CAD build for the part. Positions are in the model's coordinates, mm. A direction names the side the tool comes from. Give positions to 0.01 mm unless a question says otherwise; leave off trailing zeros. Loops run counter-clockwise (first coordinate to the right, second up) from the corner with the lowest first, then second, coordinate; pieces in that order, holes last.
Item 1: Which spindle directions (+Z, -Z, +X, -X, +Y, -Y) get a long thin tool onto all of the face, cutting with end or side? Do faces 4 (the flat face through (0, 6, 3.175)), 5 (the flat face through (-4.21, -50.79, 16.19)). Say none if no direction does.
Item 2: Saw through at C-C on y = -45.5. Give the cut face in (x, z), plus the area to 3 significant figures.
Item 3: Saw through at A-A on y = -16.75. Give the cut face in (x, z) (3 decimals), plus the area to 3 significant figures.
Item 4: Drop flat-ended pins along their axis: P1, Ø4, axis at x = 2, y = -31, coming from the -Z side; P2, Ø3, axis at x = 0, y = 0, coming from the +Z side; P3, Ø4, axis at x = 2.5, y = -48.5, coming from the -Z side; P4, Ø1, axis at x = 1.5, z = 4.5, coming from the +Y side. Give the stop position or say it passes through.
Item 5: Saw through at B-B on x = 0. Give the number of separate pieces and of enclosed holes in the cut face, plus the area to 3 significant figures.
Item 6: Mould opens along X. For faces 1 (the flat face through (-6.5, -9, 3)), 2 (the cylindrical face through (-0.961, -48.552, 16.143)), 3 (the flat face through (-2, -42, 14.578)) say: released by +X, released by -X, zero draft, split by the parting line, or undercut.
Item 7: Probe probe 1 along X at (y, z) = (-45.5, 16.5); probe 2 along X at (y, z) = (16.75, 1.65); probe 3 along Y at (x, z) = (0, 0.6). List the from-to ranges inside material, lowest first.
Autodesk Inventor part; units mm, degrees
ref_plane "YZ Plane" through (0, 0, 0) normal (1, 0, 0) x (0, 1, 0)
ref_plane "XZ Plane" through (0, 0, 0) normal (0, 1, 0) x (-1, 0, 0)
ref_plane "XY Plane" through (0, 0, 0) normal (0, 0, 1) x (1, 0, 0)
sketch "Sketch1" plane through (0, 0, 0) normal (0, 0, 1) x (1, 0, 0)
  line L0 (6.5, -25) -> (-6.5, -25)
  line L1 (-6.5, -25) -> (-6.5, 25)
  line L2 (-6.5, 25) -> (6.5, 25)
  line L3 (6.5, 25) -> (6.5, -25)
  line L4 (6.5, -25) -> (-6.5, 25) construction
  line L5 (-6.5, -25) -> (6.5, 25) construction
  line L6 (0, 16.75) -> (0, -16.75) construction
  point P0 (0, 0)
  dimension "d0" = 50
  dimension "d1" = 13
  dimension "d2" = 33.5
extrude "Plate1" add sketch "Sketch1" along normal blind 3.175
hole "Hole1" at (0, 0, 0) at (0, 16.75, 0) at (0, -16.75, 0) direction (0, 0, 1) diameter 3.3 end through all
sketch "Sketch2" plane through (6.5, -27.7496, 4.7625) normal (0, -0.8660254, -0.5) x (1, 0, 0)
  line L0 (-13, 0) -> (0, 0)
  line L1 (0, 0) -> (0, 11.3338)
  line L2 (0, 11.3338) -> (-13, 11.3338)
  line L3 (-13, 11.3338) -> (-13, 0)
edge flange "Flange1" height 15 angle 60 thickness 3.175 bend radius 3.175 thickness toward (0, -0.8660254, -0.5) relief tear relief width 3.175 relief depth 1.5875 edges at (0, -25, 3.175) wall of the first edge with corners at (-6.5, -27.7496, 4.7625) (6.5, -27.7496, 4.7625) (6.5, -33.4165, 14.5779) (-6.5, -33.4165, 14.5779)
bend "Bend1"
corner "Corner1"
sketch "Sketch3" plane through (-6.5, -38.9158, 14.5779) normal (0, 0, 1) x (1, 0, 0)
  line L0 (13, 0) -> (0, 0)
  line L1 (0, 0) -> (0, -16.3338)
  line L2 (0, -16.3338) -> (13, -16.3338)
  line L3 (13, -16.3338) -> (13, 0)
edge flange "Flange2" height 20 angle 60 thickness 3.175 bend radius 3.175 thickness toward (0, 0, 1) relief tear relief width 3.175 relief depth 1.5875 edges at (0, -36.1662, 12.9904) wall of the first edge with corners at (6.5, -38.9158, 14.5779) (-6.5, -38.9158, 14.5779) (-6.5, -55.2496, 14.5779) (6.5, -55.2496, 14.5779)
bend "Bend2"
corner "Corner2"
sketch "Sketch4" plane through (-6.5, 25, 0) normal (0, 1, 0) x (1, 0, 0)
  line L0 (0, -3.175) -> (13, -3.175)
  line L1 (13, 0) -> (13, -3.175)
  line L2 (13, 0) -> (0, 0)
  line L3 (0, 0) -> (0, -3.175)
  point P0 (6.5, 0)
extrude "Extrusion1" add sketch "Sketch4" along normal blind 12
sketch "Sketch5" plane through (-6.5, -55.2496, 17.7529) normal (0, 0, 1) x (1, 0, 0)
  circle A0 centre (6.5, 9.7496) radius 6.5
  line L0 (0, 0) -> (0, 16.3338) construction
  line L1 (0, 9.7496) -> (0, 5.4065)
  line L2 (0, 5.4065) -> (6.5, 2.7141)
  line L3 (6.5, 2.7141) -> (13, 5.4065)
  line L4 (13, 5.4065) -> (13, 9.7496)
  line L5 (13, 16.3338) -> (13, 0) construction
  line L6 (13, 16.3338) -> (0, 16.3338)
  line L7 (0, 0) -> (0, 16.3338)
  line L8 (13, 0) -> (0, 0)
  line L9 (13, 16.3338) -> (13, 0)
  point P0 (6.5, 55.2496)
  point P1 (13, 5.4065)
  point P2 (8.9874, 3.7444)
  point P3 (4.0126, 3.7444)
  point P4 (0, 5.4065)
  dimension "d33" = 45.5
  dimension "d34" = 135
extrude "Extrusion2" cut sketch "Sketch5" against normal through all contours L3 L2 A0 | L3 L9 L8 L7 L2
fillet "Fillet1" radius 1 2 edges at (-6.5, -49.8432, 16.1654) (6.5, -49.8432, 16.1654)
sketch "Sketch6" plane through (-6.5, -38.9158, 17.7529) normal (0, 0, 1) x (1, 0, 0)
  arc A0 (4.0126, -12.5894) -> (8.9874, -12.5894) centre (6.5, -6.5842) ccw
  point P0 (6.5, 38.9158)
hole "Hole2" at (0, -45.5, 17.7529) direction (0, 0, -1) diameter 6.4 end through all
equation "\"d9\" = Thickness"
equation "\"d43\" = Thickness"
equation "\"d3\" = Thickness"
equation "\"d11\" = BendReliefWidth"
equation "\"d12\" = BendReliefDepth"
equation "\"d13\" = MinimumRemnant"
equation "\"d14\" = TransitionRadius"
equation "\"d17\" = BendRadius"
equation "\"d18\" = CornerReliefSize"
equation "\"d19\" = GapSize"
equation "\"d20\" = JacobiRadiusSize"
equation "\"d21\" = BendReliefWidth"
equation "\"d22\" = BendReliefDepth"
equation "\"d23\" = MinimumRemnant"
equation "\"d24\" = TransitionRadius"
equation "\"d27\" = BendRadius"
equation "\"d28\" = CornerReliefSize"
equation "\"d29\" = GapSize"
equation "\"d30\" = JacobiRadiusSize"
equation "\"BendReliefWidth\" = Thickness"
equation "\"BendReliefDepth\" = 0.5 * Thickness"
equation "\"CornerReliefSize\" = 4 * Thickness"
equation "\"MinimumRemnant\" = 2 * Thickness"
equation "\"TransitionRadius\" = BendRadius"
equation "\"JacobiRadiusSize\" = BendRadius"
equation "\"GapSize\" = Thickness"
properties part number "Printhead Endstop Cable Guide Plate" material "Aluminum 6061"
Results below:
1. face 4: +Z, +X, -X, +Y
1. face 5: +Z, -Z, -X, -Y
2. outline: (-6.5, 14.58) - (-3.2, 14.58) - (-3.2, 17.75) - (-6.5, 17.75) - close; (3.2, 14.58) - (6.5, 14.58) - (6.5, 17.75) - (3.2, 17.75) - close
2. area: 21.0 mm2
3. outline: (-6.5, 0) - (-1.65, 0) - (-1.65, 3.175) - (-6.5, 3.175) - close; (1.65, 0) - (6.5, 0) - (6.5, 3.175) - (1.65, 3.175) - close
3. area: 30.8 mm2
4. P1: stops at z = 1.42
4. P2: passes through
4. P3: stops at z = 14.58
4. P4: stops at y = -27.13
5. separate pieces: 5
5. enclosed holes: 0
5. area: 254 mm2
6. face 1: released by -X
6. face 2: undercut
6. face 3: zero draft
7. probe 1: x = -6.5 to -3.2, 3.2 to 6.5
7. probe 2: x = -6.5 to -1.65, 1.65 to 6.5
7. probe 3: y = -27.69 to -18.4, -15.1 to -1.65, 1.65 to 15.1, 18.4 to 37
